Part model, mm, in its own coordinate system. Face numbers are marked on the shaded views. A direction names the side the tool comes from. Round coordinates to 2 decimals unless told otherwise and drop trailing zeros. Loops run counter-clockwise (first coordinate to the right, second up) from the corner with the lowest first, then second, coordinate; pieces in that order, holes last.
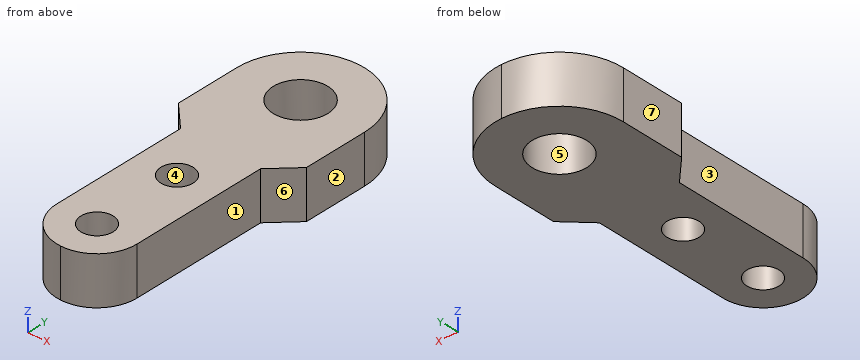
from build123d import *

# Parameters (mm, degrees)
ESQUISSE1_W             = 10
ESQUISSE1_H             = 25
BOSS_EXTRU_1_DEPTH      = 6
ESQUISSE2_W             = 16
ESQUISSE2_H             = 16
BOSS_EXTRU_2_DEPTH      = 6
ESQUISSE3_R             = 3.4
ESQUISSE3_R_2           = 2
ENL_V_MAT_EXTRU_1_DEPTH = 44.428101501
CONG_1_R                = 8
CHANFREIN1_SIZE         = 3
CONG_2_R                = 5


with BuildPart() as part:
    # Esquisse1 → Boss.-Extru.1 (new body)
    with BuildSketch(Plane.XY):
        with Locations((5, 12.5)):
            Rectangle(ESQUISSE1_W, ESQUISSE1_H)
    extrude(amount=BOSS_EXTRU_1_DEPTH)

    # Esquisse2 → Boss.-Extru.2 (add)
    with BuildSketch(Plane.XY.offset(6)):
        with Locations((5, 33)):
            Rectangle(ESQUISSE2_W, ESQUISSE2_H)
    extrude(amount=-BOSS_EXTRU_2_DEPTH)

    # Esquisse3 → Enlèv. mat.-Extru.1 (cut, through all)
    with BuildSketch(Plane.XY.offset(6)):
        with Locations((5, 33)):
            Circle(ESQUISSE3_R)
        with Locations((5, 16)):
            Circle(ESQUISSE3_R_2)
        with Locations((5, 5)):
            Circle(ESQUISSE3_R_2)
    extrude(amount=-ENL_V_MAT_EXTRU_1_DEPTH, mode=Mode.SUBTRACT)

    # Congé1
    cong_1_edges = [part.edges().sort_by_distance(p)[0] for p in [
        (13, 41, 3),
        (-3, 41, 3),
    ]]
    fillet(cong_1_edges, radius=CONG_1_R - 0.0001)  # a hair under: the kernel refuses the full size

    # Chanfrein1
    chanfrein1_edges = [part.edges().sort_by_distance(p)[0] for p in [
        (10, 25, 3),
        (0, 25, 3),
    ]]
    chamfer(chanfrein1_edges, length=CHANFREIN1_SIZE - 0.0001)  # a hair under: the kernel refuses the full size

    # Congé2
    cong_2_edges = [part.edges().sort_by_distance(p)[0] for p in [
        (10, 0, 3),
        (0, 0, 3),
    ]]
    fillet(cong_2_edges, radius=CONG_2_R - 0.0001)  # a hair under: the kernel refuses the full size


solid = part.part
1) Tool access for the marked faces 1, 2 and 3: list every direction of +Z, -Z, +X, -X, +Y, -Y with a clear straight run to the whole face (end or side of a thin tool).
Values:
face 1: +Z, -Z, +X, -Y
face 2: +Z, -Z, +X, +Y, -Y
face 3: +Z, -Z, -X, -Y
2) Wall check: line 1 along Y through (x, z) = (5, 2.95); line 2 along X through (y, z) = (7.5, 1.25); line 3 along Y through (x, z) = (3.75, 1.5). Give the ranges that are in metal, low to high.
Values:
line 1: y = 0 to 3, 7 to 14, 18 to 29.6, 36.4 to 41
line 2: x = 0 to 10
line 3: y = 0.16 to 3.44, 6.56 to 14.44, 17.56 to 29.84, 36.16 to 40.9
3) Slice it at C-C, the plane x = -1.25. Give the cut face in (y, z), then the cut area to 3 significant figures.
Values:
outline: (23.25, 0) - (37.99, 0) - (37.99, 6) - (23.25, 6) - close
area: 88.5 mm2
4) Slice it at A-A, the plane z = 5. Give the number of separate pieces and of enclosed holes in the cut face, then the cut area to 3 significant figures.
Values:
separate pieces: 1
enclosed holes: 3
area: 415 mm2
5) Drop flat-ended pins along their axis: pin 1 Ø2.5 at (x, y) = (5, 5) entering from -Z; pin 2 Ø3 at (y, z) = (5.5, 3) entering from +X; pin 3 Ø3 at (y, z) = (15, 4) entering from -X. Give the stop position or say it passes through.
Values:
pin 1: passes through
pin 2: stops at x = 10
pin 3: stops at x = 0
6) Mould opens along X. For the marked faces 4, 5, 6 and 7 say: released by +X, released by -X, zero draft, split by the parting line, or undercut.
Values:
face 4: undercut
face 5: undercut
face 6: released by +X
face 7: released by -X
7) Slice it at B-B, the plane y = 16. Give the cut face in (x, z), then the cut area to 3 significant figures.
Values:
outline: (0, 0) - (3, 0) - (3, 6) - (0, 6) - close; (7, 0) - (10, 0) - (10, 6) - (7, 6) - close
area: 36.0 mm2
8) Slice it at D-D, the plane y = 31. Give the cut face in (x, z).
Values:
outline: (-3, 0) - (2.25, 0) - (2.25, 6) - (-3, 6) - close; (7.75, 0) - (13, 0) - (13, 6) - (7.75, 6) - close
